Autodesk Inventor part; units mm, degrees
ref_plane "YZ Plane" through (0, 0, 0) normal (1, 0, 0) x (0, 1, 0)
ref_plane "XZ Plane" through (0, 0, 0) normal (0, 1, 0) x (-1, 0, 0)
ref_plane "XY Plane" through (0, 0, 0) normal (0, 0, 1) x (1, 0, 0)
sketch "Sketch1" plane through (0, 0, 0) normal (1, 0, 0) x (0, 1, 0)
  line L0 (0, 0) -> (80, 0)
  line L1 (80, 0) -> (80, -130)
  line L2 (80, -130) -> (0, -130)
  line L3 (0, -130) -> (0, 0)
  dimension "d0" = 130
  dimension "d1" = 80
extrude "Extrusion1" add sketch "Sketch1" along normal blind 30
shell "Shell1" thickness 3 removed faces 1 at (30, 53.3333, -43.3333)
sketch "Sketch2" plane through (0, 0, 0) normal (-1, 0, 0) x (0, 0, 1)
  line L0 (-127, 77) -> (-3, 77)
  line L1 (-127, 3) -> (-3, 3)
  line L2 (-127, 77) -> (-3, 77)
  line L3 (-3, 77) -> (-3, 3)
  line L4 (-3, 3) -> (-127, 3)
  line L5 (-127, 3) -> (-127, 77)
  line L6 (-65, 77) -> (-65, 41.725)
  line L7 (-127, 77) -> (-122, 77)
  line L8 (-122, 77) -> (-122, 72)
  line L9 (-122, 72) -> (-127, 72)
  line L10 (-127, 72) -> (-127, 77)
  line L11 (-3, 77) -> (-8, 77)
  line L12 (-8, 77) -> (-8, 72)
  line L13 (-8, 72) -> (-3, 72)
  line L14 (-3, 72) -> (-3, 77)
  circle A0 centre (-18.54, 72) radius 1.75
  circle A1 centre (-111.46, 72) radius 1.75
  line L15 (-111.46, 17.08) -> (-18.54, 17.08)
  circle A2 centre (-111.46, 17.08) radius 1.75
  circle A3 centre (-18.54, 17.08) radius 1.75
  line L16 (-111.46, 72) -> (-111.46, 64.54)
  line L17 (-65, 64.54) -> (-16.8, 64.54)
  line L18 (-17.8, 64.54) -> (-112.2, 64.54)
  line L19 (-113.2, 63.54) -> (-113.2, 25.14)
  line L20 (-112.2, 24.14) -> (-17.8, 24.14)
  line L21 (-16.8, 25.14) -> (-16.8, 63.54)
  arc A4 (-112.2, 64.54) -> (-113.2, 63.54) centre (-112.2, 63.54) ccw
  arc A5 (-113.2, 25.14) -> (-112.2, 24.14) centre (-112.2, 25.14) ccw
  arc A6 (-17.8, 24.14) -> (-16.8, 25.14) centre (-17.8, 25.14) ccw
  arc A7 (-16.8, 63.54) -> (-17.8, 64.54) centre (-17.8, 63.54) ccw
  point P0 (0, 0)
  point P1 (-113.2, 64.54)
  point P2 (-113.2, 24.14)
  dimension "d5" = 5
  dimension "d6" = 5
  dimension "d7" = 5
  dimension "d8" = 5
  dimension "d11" = 3.5
  dimension "d12" = 3.5
  dimension "d13" = 54.92
  dimension "d14" = 3.5
  dimension "d15" = 3.5
  dimension "d16" = 7.46
  dimension "d18" = 92.92
  dimension "d19" = 48.2
  dimension "d20" = 96.4
  dimension "d21" = 40.4
  dimension "d22" = 1
extrude "Extrusion2" cut sketch "Sketch2" against normal blind 30 contours A1 | L17 A7 L21 A6 L20 A5 L19 A4 L18 | A0 | A3 | A2
sketch "Sketch3" plane through (0, 0, 0) normal (-1, 0, 0) x (0, 0, 1)
  line L0 (-17.8, 24.14) -> (-112.2, 24.14)
  line L1 (-65, 24.14) -> (-65, 0)
  line L2 (0, 0) -> (-130, 0)
  line L3 (-65, 9.22) -> (-65, 12.07)
  line L4 (-65, 10.645) -> (-64.0682, 10.645)
  circle A0 centre (-53.2, 9.22) radius 2.85
  circle A1 centre (-29.6, 9.22) radius 2.85
  circle A2 centre (-76.8, 9.22) radius 2.85
  circle A3 centre (-100.4, 9.22) radius 2.85
  line L5 (-65, 12.07) -> (-65, 9.22)
  point P0 (-88.6, 12.07)
  point P1 (-88.6, 9.22)
extrude "Extrusion3" cut sketch "Sketch3" against normal blind 30
sketch "Sketch4" plane through (0, 80, 0) normal (0, 1, 0) x (1, 0, 0)
  line L0 (0, 130) -> (30, 130)
  circle A0 centre (15, 71.5) radius 2.5
  circle A1 centre (15, 42.5) radius 2.5
  point P0 (0, 0)
  dimension "d30" = 5
extrude "Extrusion4" cut sketch "Sketch4" against normal blind 4
properties part number "cover lcd"
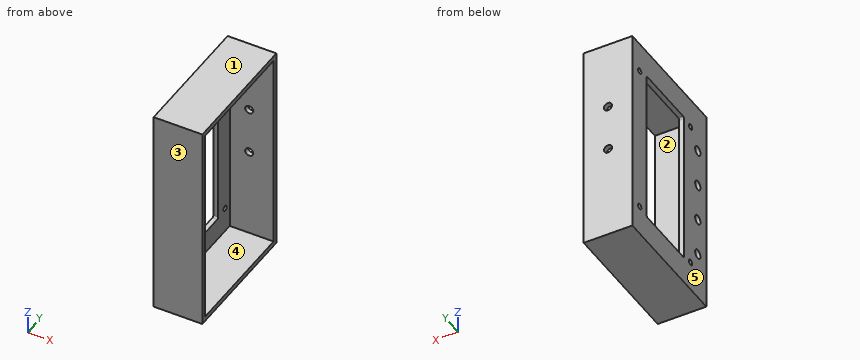
Source: CAD feature listing. Evaluate the final solid. Frame: model axes, mm. Face numbers are marked on the shaded views. A direction names the side the tool comes from. Round coordinates to 2 decimals unless told otherwise and drop trailing zeros. Loops run counter-clockwise (first coordinate to the right, second up) from the corner with the lowest first, then second, coordinate; pieces in that order, holes last. Notation, with made-up numbers: M 72,88.5 L 117,88.5 A11 ccw 117,98.5 Z; hole C 73.25,-20.75 d1. An arc over 180 degrees is marked long. Use a Markdown table: item, result. Add a question column.
1. Pull-direction query (Y, two-part tool) for the marked faces 1, 2 and 3; classes: +Y half, -Y half, draft (parallel to the pull), parting line (faces both ways), or undercut.
2. Set-up query: the marked faces 4 and 5. Return all of +Z, -Z, +X, -X, +Y, -Y with unobstructed straight access to the full face (end or side cutting, diameter ignored); none if empty.
3. Cut plane B-B, the plane z = -63. Output: boundary loops of the cut face in (x, y).
4. Cut plane D-D, the plane x = 15. Output: boundary loops of the cut face in (y, z).
5. Ray query, line 1 along Y through (x, z) = (1.2, -111.46); line 2 along Z through (x, y) = (15, 78.7); line 3 along Z through (x, y) = (4, 39.5). Return the intervals inside material, ascending. Write a range as [from, to].
6. Contact query for a flat-ended pin moving along its axis: pin 1 (10 mm diameter, centred on y = 8.5, z = -28, fed in from +X). Output: stop coordinate, or through.
7. Cut plane A-A, the plane y = 9.22. Output: boundary loops of the cut face in (x, z), and give its area (3 significant figures).
8. Cut plane C-C, the plane x = 8.75. Output: boundary loops of the cut face in (y, z).
Solution:
| question | item | result |
|---|---|---|
| 1 | face 1 | draft |
| 1 | face 2 | undercut |
| 1 | face 3 | -Y half |
| 2 | face 4 | +X |
| 2 | face 5 | +Z, -Z, -X, +Y, -Y |
| 3 | outline | M 0,0 L 30,0 L 30,3 L 3,3 L 3,24.14 L 0,24.14 Z; M 0,64.54 L 3,64.54 L 3,77 L 30,77 L 30,80 L 0,80 Z |
| 4 | outline | M 0,-130 L 80,-130 L 80,-74 L 77,-74 L 77,-127 L 3,-127 L 3,-3 L 77,-3 L 77,-40 L 80,-40 L 80,0 L 0,0 Z; M 77,-69 L 80,-69 L 80,-45 L 77,-45 Z |
| 5 | line 1 | y = [0, 15.33], [18.83, 24.14], [64.54, 70.25], [73.75, 80] |
| 5 | line 2 | z = [-130, -74], [-69, -45], [-40, 0] |
| 5 | line 3 | z = [-130, -127], [-3, 0] |
| 6 | pin 1 | stops at x = 3 |
| 7 | outline | M 0,-130 L 30,-130 L 30,-127 L 3,-127 L 3,-103.25 L 0,-103.25 Z; M 0,-97.55 L 3,-97.55 L 3,-79.65 L 0,-79.65 Z; M 0,-73.95 L 3,-73.95 L 3,-56.05 L 0,-56.05 Z; M 0,-50.35 L 3,-50.35 L 3,-32.45 L 0,-32.45 Z; M 0,-26.75 L 3,-26.75 L 3,-3 L 30,-3 L 30,0 L 0,0 Z |
| 7 | area | 484 mm2 |
| 8 | outline | M 0,-130 L 80,-130 L 80,0 L 0,0 Z; hole M 3,-127 L 77,-127 L 77,-3 L 3,-3 Z |
